```python
from build123d import *

# Parameters (mm, degrees)
BOSS_EXTRUDE1_DEPTH = 6
SKETCH2_R           = 1.25
CUT_EXTRUDE1_DEPTH  = 79.33262411
SKETCH3_R           = 1.25
CUT_EXTRUDE2_DEPTH  = 79.33262411
MOVE_FACE1_BY       = 0.08
MOVE_FACE1_2_BY     = 0.08
MOVE_FACE1_3_BY     = 0.08
MOVE_FACE1_4_BY     = 0.08
MOVE_FACE1_5_BY     = 0.08
MOVE_FACE1_6_BY     = 0.08
MOVE_FACE1_7_BY     = 0.08
MOVE_FACE1_8_BY     = 0.08
MOVE_FACE1_9_BY     = 0.08
MOVE_FACE1_10_BY    = 0.08
MOVE_FACE1_11_BY    = 0.08
MOVE_FACE1_12_BY    = 0.08
MOVE_FACE1_13_BY    = 0.08
MOVE_FACE1_14_BY    = 0.08
MOVE_FACE1_15_BY    = 0.08
MOVE_FACE1_16_BY    = 0.08
MOVE_FACE1_17_BY    = 0.08


with BuildPart() as part:
    # Sketch1 → Boss-Extrude1 (new body)
    with BuildSketch(Plane(origin=(0, 0, 0), x_dir=(1, 0, 0), z_dir=(0, 1, 0))):
        with BuildLine():
            Line((-60, 30), (-60, -30))
            ThreePointArc((-60, -30), (-54.142135624, -44.142135624), (-40, -50))
            Line((-40, -50), (40, -50))
            ThreePointArc((40, -50), (54.142135624, -44.142135624), (60, -30))
            Line((60, -30), (60, 30))
            ThreePointArc((60, 30), (54.142135624, 44.142135624), (40, 50))
            Line((40, 50), (-40, 50))
            ThreePointArc((-40, 50), (-54.142135624, 44.142135624), (-60, 30))
        make_face()
    extrude(amount=BOSS_EXTRUDE1_DEPTH)

    # Sketch2 → Cut-Extrude1 (cut, through all)
    with BuildSketch(Plane(origin=(0, 6, 0), x_dir=(1, 0, 0), z_dir=(0, 1, 0))):
        with Locations(Location((53.475, 0, 0), (0, 0, 270))):
            Circle(SKETCH2_R)
        with Locations(Location((-53.709292606, -36.227375296, 0), (0, 0, 270))):
            Circle(SKETCH2_R)
        with Locations(Location((0, 43.45, 0), (0, 0, 270))):
            Circle(SKETCH2_R)
        with Locations(Location((50.560271927, 40.506415982, 0), (0, 0, 270))):
            Circle(SKETCH2_R)
        with Locations(Location((-50.558556763, 40.508556763, 0), (0, 0, 90))):
            Circle(SKETCH2_R)
    extrude(amount=-CUT_EXTRUDE1_DEPTH, mode=Mode.SUBTRACT)

    # Sketch3 → Cut-Extrude2 (cut, through all)
    with BuildSketch(Plane(origin=(0, 6, 0), x_dir=(1, 0, 0), z_dir=(0, 1, 0))):
        with Locations(Location((-28.45, 20, 0), (0, 0, 270))):
            Circle(SKETCH3_R)
        with Locations(Location((21.55, 20, 0), (0, 0, 270))):
            Circle(SKETCH3_R)
        with Locations(Location((-28.45, -20, 0), (0, 0, 270))):
            Circle(SKETCH3_R)
        with Locations(Location((21.55, -20, 0), (0, 0, 270))):
            Circle(SKETCH3_R)
    extrude(amount=-CUT_EXTRUDE2_DEPTH, mode=Mode.SUBTRACT)

    # Move Face1: a curved face moved outward by 0.08
    add(Solid.thicken(part.faces().sort_by_distance((21.55, 3, 18.75))[0], MOVE_FACE1_BY))

    # Move Face1 2: a curved face moved outward by 0.08
    add(Solid.thicken(part.faces().sort_by_distance((54.142135624, 3, 44.142135624))[0], MOVE_FACE1_2_BY))

    # Move Face1 3: a face moved outward by 0.08
    extrude(part.faces().sort_by_distance((60, 3, 0))[0], amount=MOVE_FACE1_3_BY, dir=(1, 0, 0))

    # Move Face1 4: a curved face moved outward by 0.08
    add(Solid.thicken(part.faces().sort_by_distance((54.142135624, 3, -44.142135624))[0], MOVE_FACE1_4_BY))

    # Move Face1 5: a face moved outward by 0.08
    extrude(part.faces().sort_by_distance((0, 3, -50))[0], amount=MOVE_FACE1_5_BY, dir=(0, 0, -1))

    # Move Face1 6: a curved face moved outward by 0.08
    add(Solid.thicken(part.faces().sort_by_distance((-54.142135624, 3, -44.142135624))[0], MOVE_FACE1_6_BY))

    # Move Face1 7: a face moved outward by 0.08
    extrude(part.faces().sort_by_distance((-60, 3, 0))[0], amount=MOVE_FACE1_7_BY, dir=(-1, 0, 0))

    # Move Face1 8: a curved face moved outward by 0.08
    add(Solid.thicken(part.faces().sort_by_distance((-54.142135624, 3, 44.142135624))[0], MOVE_FACE1_8_BY))

    # Move Face1 9: a face moved outward by 0.08
    extrude(part.faces().sort_by_distance((0, 3, 50))[0], amount=MOVE_FACE1_9_BY, dir=(0, 0, 1))

    # Move Face1 10: a curved face moved outward by 0.08
    add(Solid.thicken(part.faces().sort_by_distance((53.475, 3, -1.25))[0], MOVE_FACE1_10_BY))

    # Move Face1 11: a curved face moved outward by 0.08
    add(Solid.thicken(part.faces().sort_by_distance((0, 3, -44.7))[0], MOVE_FACE1_11_BY))

    # Move Face1 12: a curved face moved outward by 0.08
    add(Solid.thicken(part.faces().sort_by_distance((50.560271927, 3, -41.756415982))[0], MOVE_FACE1_12_BY))

    # Move Face1 13: a curved face moved outward by 0.08
    add(Solid.thicken(part.faces().sort_by_distance((-50.558556763, 3, -39.258556763))[0], MOVE_FACE1_13_BY))

    # Move Face1 14: a curved face moved outward by 0.08
    add(Solid.thicken(part.faces().sort_by_distance((-53.709292606, 3, 34.977375296))[0], MOVE_FACE1_14_BY))

    # Move Face1 15: a curved face moved outward by 0.08
    add(Solid.thicken(part.faces().sort_by_distance((-28.45, 3, -21.25))[0], MOVE_FACE1_15_BY))

    # Move Face1 16: a curved face moved outward by 0.08
    add(Solid.thicken(part.faces().sort_by_distance((21.55, 3, -21.25))[0], MOVE_FACE1_16_BY))

    # Move Face1 17: a curved face moved outward by 0.08
    add(Solid.thicken(part.faces().sort_by_distance((-28.45, 3, 18.75))[0], MOVE_FACE1_17_BY))


solid = part.part
```
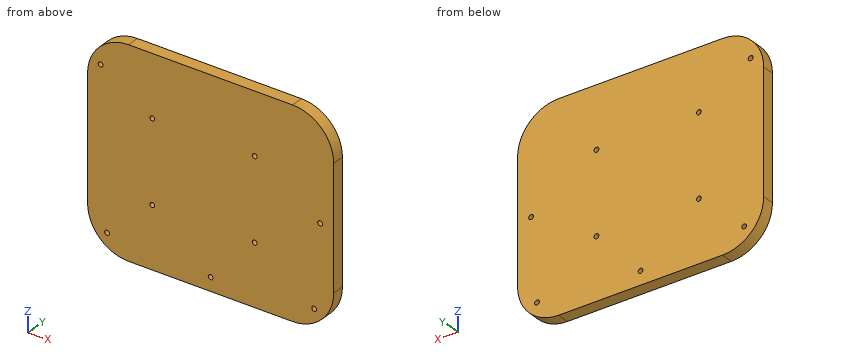
For this review, take the finished solid that the model builds, in its own axes (mm). Coordinates: 2 decimals unless noted, no trailing zeros. Put each result on its own line as item: value.
1. For pin 1 (1.4 mm diameter, centred on x = -28.45, z = -20, fed in from -Y); pin 2 (1 mm diameter, centred on y = 3.5, z = -34.5, fed in from +X); pin 3 (3 mm diameter, centred on x = 53.475, z = 0, fed in from +Y), all flat-tipped, find the tip position at first contact; note any pin that passes through.
Values found:
pin 1: through
pin 2: x = 59.68
pin 3: y = 6
2. Add section A-A, the plane y = 2.2. Count the separate pieces of the cut face and the enclosed holes in it, then the cut area to 3 significant figures.
Values found:
separate pieces: 1
enclosed holes: 9
area: 11,700 mm²
3. Wall thickness on probe 1 along X at (y, z) = (3.95, -20); probe 2 along X at (y, z) = (5, -20.5); probe 3 along Z at (x, y) = (-53, 1): over which ranges is each line inside the solid? List them lowest first.
Values found:
probe 1: -60.08 to -29.62, -27.28 to 20.38, 22.72 to 60.08
probe 2: -60.08 to -29.51, -27.39 to 20.49, 22.61 to 60.08
probe 3: -45.3 to 35.3, 37.16 to 45.3
